from build123d import *

# Parameters (mm, degrees)
SKETCH016_W             = 31.3
SKETCH016_H             = 14.4
PAD007_DEPTH            = 1.6
SKETCH017_R             = 1.5
POCKET006_DEPTH         = 1.6
SKETCH018_W             = 6
SKETCH018_H             = 13.2
PAD008_DEPTH            = 10.2
SKETCH019_W             = 6
SKETCH019_H             = 5
POCKET007_DEPTH         = 8.1
BODY004_PLACEMENT_ANGLE = 180


with BuildPart() as part:
    # Sketch016 → Pad007 (new body)
    with BuildSketch(Plane.XY.offset(-1.6)):
        with Locations((15.65, 7.2)):
            Rectangle(SKETCH016_W, SKETCH016_H)
    extrude(amount=PAD007_DEPTH)

    # Sketch017 (on Face6 of Pad007) → Pocket006 (cut)
    with BuildSketch(Plane.XY):
        with Locations((24.4, 7.2)):
            Circle(SKETCH017_R)
    extrude(amount=-POCKET006_DEPTH, mode=Mode.SUBTRACT)

    # Sketch018 (on Face5 of Pocket006) → Pad008 (join)
    with BuildSketch(Plane.XY):
        with Locations((3.85, 6.6)):
            Rectangle(SKETCH018_W, SKETCH018_H)
    extrude(amount=PAD008_DEPTH)

    # Sketch019 (on Face12 of Pad008) → Pocket007 (cut)
    with BuildSketch(Plane.XY.offset(10.2)):
        with Locations((3.85, 6.55)):
            Rectangle(SKETCH019_W, SKETCH019_H)
    extrude(amount=-POCKET007_DEPTH, mode=Mode.SUBTRACT)


with BuildPart() as part_1:
    # Body004 placement: moved
    add(part.part.moved(Location((13.5, -15, 1.5))).rotate(Axis((13.5, -15, 1.5), (0, 0, 1)), BODY004_PLACEMENT_ANGLE))


solid = part_1.part
Can you work these out from the model? Positions are in its coordinate system, mm. A direction names the side the tool comes from. Give positions to 0.01 mm unless a question says otherwise; leave off trailing zeros. Write each loop counter-clockwise with the first axis right and the second up, starting at its lowest first coordinate (ties: lowest second). Pieces come first, ordered by that corner, then holes. Notation, with made-up numbers: M 73,28.5 L 123,28.5 A33 ccw 123,61.5 Z; hole C -17.5,-15 d11. An arc over 180 degrees is marked long. Answer in a Markdown table with one row per item. Add a question column.
Item 1: Imagine slicing it at A-A, the plane x = -10. Write out the boundary of the cut face in (y, z).
Item 2: Imagine slicing it at D-D, the plane y = -19.5. Write out the boundary of the cut face in (x, z).
Item 3: Imagine slicing it at C-C, the plane z = 8.5. Write out the boundary of the cut face in (x, y).
Item 4: On a 3-axis mill with a long thin cutter (end or side, diameter ignored), from which of +Z, -Z, +X, -X, +Y, -Y can I reach the whole of each face in a straight line? I mean faces 4 (the flat face through (10, -24.05, 8)), 5 (the flat face through (10, -28.2, 7)), 6 (the flat face through (13.5, -22, 1)), 7 (the flat face through (12.65, -24.4, 6.5)). Say none if no direction works.
Item 5: For pin 1 Ø5 at (y, z) = (-17, 5) entering from +X; pin 2 Ø6.5 at (x, z) = (10, 6.5) entering from -Y; pin 3 Ø2.5 at (x, y) = (8.5, -21.5) entering from +Z, each with a flat end and sliding along its axis, tell me the tip position at first contact or that it passes through.
Item 6: Please list where these lines run through material, in increasing order: L1, parallel to Y at x = 10, z = 9.25; L2, parallel to Y at x = -10.9, z = 1.05; L3, parallel to X at y = -15.75, z = 7.
Item 7: We'd pull the mould along X, two halves only. Please class faces 1 (the cylindrical face through (-9.79, -23.21, 0.71)), 2 (the flat face through (6.65, -24.4, 6.5)), 3 (the flat face through (10, -26, 11.7)): released by +X, released by -X, zero draft, split by the parting line, or undercut.
Item 8: Imagine slicing it at B-B, the plane y = -22.2. Write out the boundary of the cut face in (x, z), plus the area to 3 significant figures.
Evaluation:
| question | item | result |
|---|---|---|
| 1 | outline | M -29.4,-0.1 L -23.4,-0.1 L -23.4,1.5 L -29.4,1.5 Z; M -21,-0.1 L -15,-0.1 L -15,1.5 L -21,1.5 Z |
| 2 | outline | M -17.8,-0.1 L 13.5,-0.1 L 13.5,1.5 L 12.65,1.5 L 12.65,3.6 L 6.65,3.6 L 6.65,1.5 L -17.8,1.5 Z |
| 3 | outline | M 6.65,-28.2 L 12.65,-28.2 L 12.65,-24.05 L 6.65,-24.05 Z; M 6.65,-19.05 L 12.65,-19.05 L 12.65,-15 L 6.65,-15 Z |
| 4 | face 4 | +Z, +X, -X |
| 4 | face 5 | +Z, +X, -X, -Y |
| 4 | face 6 | +Z, -Z, +X, +Y, -Y |
| 4 | face 7 | +Z, +X, +Y, -Y |
| 5 | pin 1 | stops at x = 12.65 |
| 5 | pin 2 | stops at y = -28.2 |
| 5 | pin 3 | stops at z = 3.6 |
| 6 | L1 | y = -28.2 to -24.05, -19.05 to -15 |
| 6 | L2 | y = -29.4 to -23.7, -20.7 to -15 |
| 6 | L3 | x = 6.65 to 12.65 |
| 7 | face 1 | undercut |
| 7 | face 2 | released by -X |
| 7 | face 3 | zero draft |
| 8 | outline | M -17.8,-0.1 L -12.4,-0.1 L -12.4,1.5 L -17.8,1.5 Z; M -9.4,-0.1 L 13.5,-0.1 L 13.5,1.5 L 12.65,1.5 L 12.65,3.6 L 6.65,3.6 L 6.65,1.5 L -9.4,1.5 Z |
| 8 | area | 57.9 mm² |
